```python
from build123d import *

# Parameters (mm, degrees)
SKETCH1_W           = 173
SKETCH1_H           = 64
BOSS_EXTRUDE1_DEPTH = 29
SHELL1_T            = -2
SKETCH3_W           = 2
SKETCH3_H           = 60
BOSS_EXTRUDE2_DEPTH = 27


with BuildPart() as part:
    # Sketch1 → Boss-Extrude1 (new body)
    with BuildSketch(Plane(origin=(0, 0, 0), x_dir=(1, 0, 0), z_dir=(0, 1, 0))):
        Rectangle(SKETCH1_W, SKETCH1_H)
    extrude(amount=BOSS_EXTRUDE1_DEPTH)

    # Shell1
    shell1_openings = [part.faces().sort_by_distance(p)[0] for p in [
        (0, 29, 0),
    ]]
    offset(amount=SHELL1_T, openings=shell1_openings, kind=Kind.INTERSECTION)

    # Sketch3 → Boss-Extrude2 (add)
    with BuildSketch(Plane(origin=(0, 2, 0), x_dir=(1, 0, 0), z_dir=(0, 1, 0))):
        with Locations((-33.5, 0)):
            Rectangle(SKETCH3_W, SKETCH3_H)
    extrude(amount=BOSS_EXTRUDE2_DEPTH)


solid = part.part
```
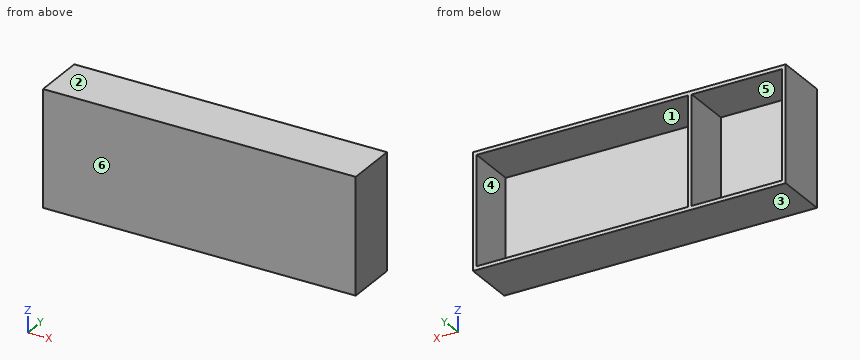
Geometry: final body of the model. Coordinates: model frame, mm. Face numbers are marked on the shaded views. A direction names the side the tool comes from. Round coordinates to 2 decimals unless told otherwise and drop trailing zeros. Loops run counter-clockwise (first coordinate to the right, second up) from the corner with the lowest first, then second, coordinate; pieces in that order, holes last.
Item 1: Section A-A, the plane y = 3.75. Output: boundary loops of the cut face in (x, z).
Checked values:
outline: (-86.5, -32) - (86.5, -32) - (86.5, 32) - (-86.5, 32) - close; hole (-84.5, -30) - (-34.5, -30) - (-34.5, 30) - (-84.5, 30) - close; hole (-32.5, -30) - (84.5, -30) - (84.5, 30) - (-32.5, 30) - close
Item 2: Contact query for flat-ended pins moving along their axis: P1, Ø15, axis at x = -47.5, z = -7.5, coming from the +Y side; P2, Ø1, axis at x = -42, z = -18, coming from the -Y side. Output: stop coordinate, or through.
Checked values:
P1: stops at y = 2
P2: stops at y = 0
Item 3: Section B-B, the plane x = -36. Output: boundary loops of the cut face in (y, z).
Checked values:
outline: (0, -32) - (29, -32) - (29, -30) - (2, -30) - (2, 30) - (29, 30) - (29, 32) - (0, 32) - close
Item 4: Section C-C, the plane z = -15. Output: boundary loops of the cut face in (x, y).
Checked values:
outline: (-86.5, 0) - (86.5, 0) - (86.5, 29) - (84.5, 29) - (84.5, 2) - (-32.5, 2) - (-32.5, 29) - (-34.5, 29) - (-34.5, 2) - (-84.5, 2) - (-84.5, 29) - (-86.5, 29) - close
Item 5: Mould query, pull axis Z, two halves, no side actions, for the marked faces 1, 2, 3 and 4. Classes: released by +Z, released by -Z, zero draft, split by the parting line, or undercut.
Checked values:
face 1: undercut
face 2: released by +Z
face 3: released by -Z
face 4: undercut
Item 6: Reachability of the marked faces 5 and 6 from +Z, -Z, +X, -X, +Y, -Y: full face, straight path, thin tool, end or side. Return the list, or none.
Checked values:
face 5: +Y
face 6: +Z, -Z, +X, -X, -Y
Item 7: Line query: L1, parallel to X at y = 19, z = -26.5; L2, parallel to Z at x = 14.5, y = 6.5; L3, parallel to Y at x = -57, z = -10.5. Output: solid intervals per line, ascending.
Checked values:
L1: x = -86.5 to -84.5, -34.5 to -32.5, 84.5 to 86.5
L2: z = -32 to -30, 30 to 32
L3: y = 0 to 2
